The listing builds one solid part. Answer for the finished solid, in the listing's coordinates (mm). A direction names the side the tool comes from. Round coordinates to 2 decimals unless told otherwise and drop trailing zeros. Order: outer loops, then holes, each group sorted by start corner. A loop starts at its lowest first (then second) coordinate and runs counter-clockwise, first axis right, second up. Notation, with made-up numbers: M -23.5,70.25 L -18.5,70.25 A21 ccw -18.5,74.25 Z; hole C -7.75,-21.5 d1. An arc over 180 degrees is marked long. Put each result on its own line as item: value. Start each with the question number.
1. The mould has two halves that part along X. Classify faces 1 (the face through (0, 11, 0)), 2 (the face through (-4, 19, -3)), 3 (the face through (-12, 3, -15)), 4 (the face through (-15, 5, -9)): +X half, -X half, draft (parallel to the pull), parting line (faces both ways), or undercut.
2. The part is cut by section B-B (z = -15). Give the vertices of the cut face in (x, y).
3. Each of these flat-tipped pins is pushed along its axis until it touches: pin 1 Ø3.5 at (x, z) = (10, -15) entering from -Y; pin 2 Ø10 at (x, y) = (-3.5, 26) entering from -Z. Where does it stop, or does it pass through?
4. The part is cut by section C-C (x = 10). Give the vertices of the cut face in (y, z).
5. The part is cut by section A-A (y = 19.25). Give the vertices of the cut face in (x, z), then the cut area to 3 significant figures.
6. The part is cut by section D-D (z = -3). Give the vertices of the cut face in (x, y), then the cut area to 3 significant figures.
7. Which of the six approach directions +Z, -Z, +X, -X, +Y, -Y give full straight-line access (tool end or side, diameter ignored) to faces 5 (the face through (15, 5, -9)), 6 (the face through (4, 15, -6)), 7 (the face through (0, 24, -3))?
8. Consider line 1 (X direction, y = 3.1, z = -15); line 2 (Z direction, x = -10, y = 2.35); line 3 (Z direction, x = -3, y = 11). Determine where each line is inside the solid, lowest interval first.
from build123d import *

# Parameters (mm, degrees)
EXTRUDE_1_DEPTH     = 15
SKETCH_2_R          = 2
CUT_EXTRUDE_1_DEPTH = 40
CUT_EXTRUDE_2_DEPTH = 40


with BuildPart() as part:
    # 草图1 → 凸台-拉伸1 (new, symmetric)
    with BuildSketch(Plane(origin=(0, 0, 0), x_dir=(0, 0, -1), z_dir=(1, 0, 0))):
        Polygon((0, 0), (0, 29), (6, 29), (6, 6), (30, 6), (30, 0), align=None)
    extrude(amount=EXTRUDE_1_DEPTH, both=True)

    # 草图2 → 切除-拉伸1 (cut)
    with BuildSketch(Plane(origin=(0, 0, 0), x_dir=(1, 0, 0), z_dir=(0, 1, 0))):
        with Locations(Location((-10, 15, 0), (0, 0, 90))):
            Circle(SKETCH_2_R)
        with Locations(Location((10, 15, 0), (0, 0, 90))):
            Circle(SKETCH_2_R)
    extrude(amount=CUT_EXTRUDE_1_DEPTH, mode=Mode.SUBTRACT)

    # 草图3 → 切除-拉伸2 (cut)
    with BuildSketch(Plane.XY):
        with BuildLine():
            Line((-4, 22), (-4, 16))
            ThreePointArc((-4, 16), (0, 14), (4, 16))
            Line((4, 16), (4, 22))
            ThreePointArc((4, 22), (0, 24), (-4, 22))
        make_face()
    extrude(amount=-CUT_EXTRUDE_2_DEPTH, mode=Mode.SUBTRACT)


solid = part.part
Resolved:
1. face 1: draft
1. face 2: undercut
1. face 3: undercut
1. face 4: -X half
2. outline: M -15,0 L -12,0 L -12,6 L -15,6 Z; M -8,0 L 8,0 L 8,6 L -8,6 Z; M 12,0 L 15,0 L 15,6 L 12,6 Z
3. pin 1: through
3. pin 2: z = -6
4. outline: M 0,-30 L 6,-30 L 6,-17 L 0,-17 Z; M 0,-13 L 6,-13 L 6,-6 L 29,-6 L 29,0 L 0,0 Z
5. outline: M -15,-6 L -4,-6 L -4,0 L -15,0 Z; M 4,-6 L 15,-6 L 15,0 L 4,0 Z
5. area: 132 mm2
6. outline: M -15,0 L 15,0 L 15,29 L -15,29 Z; hole M -4,16 A5 ccw 4,16 L 4,22 A5 ccw -4,22 Z
6. area: 800 mm2
7. face 5: +Z, -Z, +X, +Y, -Y
7. face 6: -Z, +X, -X, +Y
7. face 7: +Z, -Z
8. line 1: -15 to -12, -8 to 8, 12 to 15
8. line 2: -30 to -17, -13 to 0
8. line 3: -6 to 0
